```python
from build123d import *

# Parameters (mm, degrees)
F1_DEPTH = 2


with BuildPart() as f1:
    # F0 (on Front) → F1 (new body)
    with BuildSketch(Plane.XZ):
        with BuildLine():
            ThreePointArc((-38.4432851938, 37.1302077967), (-41.8189272985, 31.7253624753), (-40.6708321656, 25.4572534994))
            Line((-40.6708321656, 25.4572534994), (-40.6635933433, 25.4572770938))
            Line((-40.6635933433, 25.4572770938), (-37.9443538187, 25.4661402565))
            ThreePointArc((-37.9443538187, 25.4661402565), (-39.7897986845, 29.6891767659), (-38.4432851938, 34.0967390777))
            Line((-38.4432851938, 34.0967390777), (-38.4432851938, 37.1302077967))
        make_face()
        with BuildLine():
            ThreePointArc((-24.3404475114, 30.0725679845), (-24.9999427639, 33.418477972), (-26.8797747894, 36.2638741112))
            Line((-26.8797747894, 36.2638741112), (-27.1338318028, 32.8728124835))
            ThreePointArc((-27.1338318028, 32.8728124835), (-26.6713997999, 31.5064940955), (-26.5147945554, 30.0725679845))
            ThreePointArc((-26.5147945554, 30.0725679845), (-26.9883189893, 27.6094284081), (-28.3413854132, 25.4974404311))
            Line((-28.3413854132, 25.4974404311), (-25.6149070662, 25.5063271883))
            ThreePointArc((-25.6149070662, 25.5063271883), (-24.6650368609, 27.7021881539), (-24.3404475114, 30.0725679845))
        make_face()
        with BuildLine():
            Line((-28.3413854132, 25.4974404311), (-29.3841796517, 22.103513683))
            ThreePointArc((-29.3841796517, 22.103513683), (-27.2492776233, 23.5277028406), (-25.6149070662, 25.5063271883))
            Line((-25.6149070662, 25.5063271883), (-28.3413854132, 25.4974404311))
        make_face()
        with BuildLine():
            Line((-40.6610403277, 25.4482014486), (-40.6575024619, 25.4356247862))
            ThreePointArc((-40.6575024619, 25.4356247862), (-39.1888748371, 23.6403973669), (-37.3029250496, 22.2902484912))
            Line((-37.3029250496, 22.2902484912), (-37.9443538187, 25.4661402565))
            Line((-37.9443538187, 25.4661402565), (-40.6635933433, 25.4572770938))
            Line((-40.6635933433, 25.4572770938), (-40.6610403277, 25.4482014486))
        make_face()
        with BuildLine():
            Line((-40.6575024619, 25.4356247862), (-38.1070154905, 16.368968524))
            Line((-38.1070154905, 16.368968524), (-36.1070154905, 16.368968524))
            Line((-36.1070154905, 16.368968524), (-37.3029250496, 22.2902484912))
            ThreePointArc((-37.3029250496, 22.2902484912), (-39.1888748371, 23.6403973669), (-40.6575024619, 25.4356247862))
        make_face()
        with BuildLine():
            Line((-44.1070154905, 16.368968524), (-45.6070154905, 16.368968524))
            Line((-45.6070154905, 16.368968524), (-45.6070154905, 14.368968524))
            Line((-45.6070154905, 14.368968524), (-33.6070154905, 14.368968524))
            Line((-33.6070154905, 14.368968524), (-33.6070154905, 13.368968524))
            Line((-33.6070154905, 13.368968524), (-45.6070154905, 13.368968524))
            Line((-45.6070154905, 13.368968524), (-45.6070154905, 11.368968524))
            Line((-45.6070154905, 11.368968524), (-44.1070154905, 11.368968524))
            Line((-44.1070154905, 11.368968524), (-44.1070154905, 11.868968524))
            Line((-44.1070154905, 11.868968524), (-41.6070154905, 11.868968524))
            Line((-41.6070154905, 11.868968524), (-41.6070154905, 11.368968524))
            Line((-41.6070154905, 11.368968524), (-32.6070154905, 11.368968524))
            Line((-32.6070154905, 11.368968524), (-32.6070154905, 13.368968524))
            Line((-32.6070154905, 13.368968524), (-32.1070154905, 13.368968524))
            Line((-32.1070154905, 13.368968524), (-32.1070154905, 11.368968524))
            Line((-32.1070154905, 11.368968524), (-28.1070154905, 11.368968524))
            Line((-28.1070154905, 11.368968524), (-25.6149070662, 25.5063271883))
            ThreePointArc((-25.6149070662, 25.5063271883), (-27.2492776233, 23.5277028406), (-29.3841796517, 22.103513683))
            Line((-29.3841796517, 22.103513683), (-31.6070154905, 14.868968524))
            Line((-31.6070154905, 14.868968524), (-31.6070154905, 16.368968524))
            Line((-31.6070154905, 16.368968524), (-33.6070154905, 16.368968524))
            Line((-33.6070154905, 16.368968524), (-36.1070154905, 16.368968524))
            Line((-36.1070154905, 16.368968524), (-38.1070154905, 16.368968524))
            Line((-38.1070154905, 16.368968524), (-41.6070154905, 16.368968524))
            Line((-41.6070154905, 16.368968524), (-41.6070154905, 15.868968524))
            Line((-41.6070154905, 15.868968524), (-44.1070154905, 15.868968524))
            Line((-44.1070154905, 15.868968524), (-44.1070154905, 16.368968524))
        make_face()
    extrude(amount=F1_DEPTH)


solid = f1.part
```
Could you check a few things on this model? Use its own coordinates, in mm. A direction names the side the tool comes from. Coordinates: 2 decimals unless noted, no trailing zeros. Write each loop counter-clockwise with the first axis right and the second up, starting at its lowest first coordinate (ties: lowest second). Pieces come first, ordered by that corner, then holes. Notation, with made-up numbers: (-2.75, -10) -> (55.25, -10) arc R15 ccw to (55.25, 14) -> close; hole circle Ø8 at (-5, 68). An arc over 180 degrees is marked (long way). Return JSON: item names as keys, results as strings.
(1) I need wall thicknesses on L1, parallel to Z at x = -41.25, y = -1.3; L2, parallel to Z at x = -32.5, y = -1.35; L3, parallel to X at y = -1.6, z = 27. Which ranges of each line are inside material? Lowest first, please.
Numbers:
{"L1": "z = 11.37 to 13.37, 14.37 to 16.37, 26.57 to 33.57", "L2": "z = 13.37 to 16.37", "L3": "x = -41.42 to -39.05, -27.27 to -24.89"}
(2) Imagine slicing it at D-D, the plane x = -27.75. Please give me the cut outline in (y, z), then the cut area to 3 significant figures.
Numbers:
{"outline": "(-2, 13.39) -> (0, 13.39) -> (0, 26.21) -> (-2, 26.21) -> close", "area": "25.6 mm2"}
(3) I'm going to push flat-ended pins straight in: pin 1 (1 mm diameter, centred on x = -40.5, y = -1, fed in from +Z); pin 2 (0.6 mm diameter, centred on x = -41, y = -1, fed in from +Z); pin 3 (0.6 mm diameter, centred on x = -33, y = -1, fed in from +Z). Where does each tip first touch, or does it pass through?
Numbers:
{"pin 1": "stops at z = 35.63", "pin 2": "stops at z = 34.64", "pin 3": "stops at z = 16.37"}
(4) Imagine slicing it at A-A, the plane x = -44.5. Please give me the cut outline in (y, z).
Numbers:
{"outline": "(-2, 11.37) -> (0, 11.37) -> (0, 13.37) -> (-2, 13.37) -> close; (-2, 14.37) -> (0, 14.37) -> (0, 16.37) -> (-2, 16.37) -> close"}
(5) Imagine slicing it at B-B, the plane z = 18. Please give me the cut outline in (x, y) (3 decimals), then the cut area to 3 significant figures.
Numbers:
{"outline": "(-38.566, -2) -> (-36.436, -2) -> (-36.436, 0) -> (-38.566, 0) -> close; (-30.645, -2) -> (-26.938, -2) -> (-26.938, 0) -> (-30.645, 0) -> close", "area": "11.7 mm2"}
(6) Which directions (+Z, -Z, +X, -X, +Y, -Y) give clear straight access to the entire face, cutting with the end or side of a thin tool? Please do faces 1 (the flat face through (-32.107, -1, 12)), 2 (the flat face through (-38.443, -1, 36)), 3 (the cylindrical face through (-39.786, -0.986, 29.623)), 4 (the flat face through (-40, -1, 13.369)).
Numbers:
{"face 1": "-Z, +Y, -Y", "face 2": "+Z, +Y, -Y", "face 3": "+Y, -Y", "face 4": "-X, +Y, -Y"}
(7) Imagine slicing it at C-C, the plane x = -39.5. Please give me the cut outline in (y, z), then the cut area to 3 significant figures.
Numbers:
{"outline": "(-2, 11.37) -> (0, 11.37) -> (0, 13.37) -> (-2, 13.37) -> close; (-2, 14.37) -> (0, 14.37) -> (0, 16.37) -> (-2, 16.37) -> close; (-2, 21.32) -> (0, 21.32) -> (0, 28.1) -> (-2, 28.1) -> close; (-2, 32.05) -> (0, 32.05) -> (0, 36.2) -> (-2, 36.2) -> close", "area": "29.8 mm2"}
